Source: CAD feature listing. Evaluate the final solid. Frame: model axes, mm. A direction names the side the tool comes from. Give positions to 0.01 mm unless a question says otherwise; leave off trailing zeros. Order: outer loops, then holes, each group sorted by start corner. A loop starts at its lowest first (then second) coordinate and runs counter-clockwise, first axis right, second up. Notation, with made-up numbers: M 2.25,-25.75 L 14.25,-25.75 A30 cw 14.25,3.25 Z; hole C -23,2.5 d4. An arc over 180 degrees is marked long. Answer in a Markdown table with one row per item. Add a question column.
(1) Section query A-A, the plane y = 9.66. Return loops of the section in (x, z) (3 decimals).
(2) Mould query, pull axis X, two halves, no side actions, for faces 1 (the face through (-0.063, 10.142, 14.232)), 2 (the face through (-4.668, 2.401, -2.745)), 3 (the face through (4.668, 2.401, 2.745)). Classes: pulls with the +X half, pulls with the -X half, needs draft (parallel to the pull), parting line crosses it, or undercut.
(3) Section query C-C, the plane x = -2.5. Return loops of the section in (y, z) (3 decimals).
(4) Section query B-B, the plane z = 8. Return loops of the section in (x, y) (3 decimals), plus the area to 3 significant figures.
(5) Pin query (flat end, axial travel): P1, Ø5.5, axis at x = 1, y = 1.5, coming from the +Z side (3 decimals); P2, Ø2, axis at x = -3.5, z = 18, coming from the -Y side; P3, Ø1.5, axis at y = 2, z = 4.5, coming from the -X side; P4, Ø1.5, axis at x = 0, z = 4, coming from the -Y side. Return the tip coordinate at first contact, or that it passes through.
(6) Section query D-D, the plane y = 0.75. Return loops of the section in (x, z) (3 decimals), plus the area to 3 significant figures.
(7) Set-up query: faces 4 (the face through (2.388, 9.011, -4.165)), 5 (the face through (1.33, -0.25, -2.56)), 6 (the face through (0, 4.87, 6)), 7 (the face through (-5.4, 4.87, -0.3)), 8 (the face through (0, 2, 5.415)). Return all of +Z, -Z, +X, -X, +Y, -Y with unobstructed straight access to the full face (end or side cutting, diameter ignored); none if empty.
(8) Material intervals for line 1 along Y through (x, z) = (0, 13) (3 decimals); line 2 along Y through (x, z) = (3.5, 0.75); line 3 along Z through (x, y) = (-0.25, 3) (3 decimals), sorted ascending.
from build123d import *

# Parameters (mm, degrees)
BOSS_EXTRUDE1_DEPTH = 4.87
BOSS_EXTRUDE2_DEPTH = 8.4
SKETCH3_R           = 1.115
SKETCH3_R_2         = 0.48582374
BOSS_EXTRUDE3_DEPTH = 15
SKETCH4_R           = 2.886437974
BOSS_EXTRUDE4_DEPTH = 0.5


with BuildPart() as part:
    # Sketch1 → Boss-Extrude1 (new body)
    with BuildSketch(Plane(origin=(0, 0, 0), x_dir=(1, 0, 0), z_dir=(0, 1, 0))):
        Polygon((6.252703415, 0), (3.126351708, 5.415), (-3.126351708, 5.415), (-6.252703415, 0), (-3.126351708, -5.415), (3.126351708, -5.415), align=None)
    extrude(amount=BOSS_EXTRUDE1_DEPTH)

    # Sketch2 → Boss-Extrude2 (add)
    with BuildSketch(Plane(origin=(0, 4.87, 0), x_dir=(1, 0, 0), z_dir=(0, 1, 0))):
        Polygon((0, 5.065814818), (-4.710329867, 3.289588054), (-5.5, -6.837347299), (-1.528536321, -6.837347299), (5.5, -6.837347299), (4.710329867, 3.289588054), align=None)
    extrude(amount=BOSS_EXTRUDE2_DEPTH)

    # Sketch3 → Boss-Extrude3 (add)
    with BuildSketch(Plane.XY.offset(6.837347299)):
        with Locations((0, 9.66)):
            Circle(SKETCH3_R)
        with Locations((0, 9.66)):
            Circle(SKETCH3_R_2, mode=Mode.SUBTRACT)
    extrude(amount=BOSS_EXTRUDE3_DEPTH)

    # Sketch4 → Boss-Extrude4 (add)
    with BuildSketch(Plane.XZ):
        Circle(SKETCH4_R)
    extrude(amount=BOSS_EXTRUDE4_DEPTH)


solid = part.part
Values follow:
| question | item | result |
|---|---|---|
| 1 | outline | M -5.5,6.837 L -4.71,-3.29 L 0,-5.066 L 4.71,-3.29 L 5.5,6.837 L 1.115,6.837 L 1.115,21.837 L 0.486,21.837 L 0.486,6.837 L -0.486,6.837 L -0.486,21.837 L -1.115,21.837 L -1.115,6.837 Z |
| 2 | face 1 | undercut |
| 2 | face 2 | pulls with the -X half |
| 2 | face 3 | pulls with the +X half |
| 3 | outline | M -0.5,-1.443 L 0,-1.443 L 0,-5.415 L 4.87,-5.415 L 4.87,-4.123 L 13.27,-4.123 L 13.27,6.837 L 4.87,6.837 L 4.87,5.415 L 0,5.415 L 0,1.443 L -0.5,1.443 Z |
| 4 | outline | C 0,9.66 d2.23; hole C 0,9.66 d0.972 |
| 4 | area | 3.16 mm² |
| 5 | P1 | stops at z = 5.415 |
| 5 | P2 | passes through |
| 5 | P3 | stops at x = -4.09 |
| 5 | P4 | stops at y = 0 |
| 6 | outline | M -6.253,0 L -3.126,-5.415 L 3.126,-5.415 L 6.253,0 L 3.126,5.415 L -3.126,5.415 Z |
| 6 | area | 102 mm² |
| 7 | face 4 | -Z, +X, +Y |
| 7 | face 5 | -Y |
| 7 | face 6 | +Z, -Y |
| 7 | face 7 | -Z, -X, +Y |
| 7 | face 8 | +Z, +X, -X, -Y |
| 8 | line 1 | y = 8.545 to 9.174, 10.146 to 10.775 |
| 8 | line 2 | y = 0 to 13.27 |
| 8 | line 3 | z = -5.415 to 5.415 |
